Input: part model. Units: mm. Frame: model coordinates. A direction names the side the tool comes from. Coordinates: 2 decimals unless noted, no trailing zeros. Write each loop counter-clockwise with the first axis right and the second up, starting at its lowest first coordinate (ties: lowest second). Pieces come first, ordered by that corner, then holes. Notation, with made-up numbers: M -23.75,82.5 L -0.75,82.5 A16 ccw -0.75,105.5 Z; hole C 15.5,56.5 d3. An arc over 180 degrees is marked long. Answer as a JSON object with one key per item and string values. Group by question number.
from build123d import *

# Parameters (mm, degrees)
BOSS_EXTRUDE1_DEPTH = 13
BOSS_EXTRUDE3_DEPTH = 2.3
BOSS_EXTRUDE4_DEPTH = 2.3
SPLIT1_START        = -4.6
SPLIT1_DEPTH        = 4.6
SKETCH9_W           = 56.929943861
SKETCH9_H           = 73.17042397
BOSS_EXTRUDE5_DEPTH = 34
SKETCH10_W          = 56
SKETCH10_H          = 74
SKETCH10_W_2        = 52
SKETCH10_H_2        = 70
BOSS_EXTRUDE6_DEPTH = 10
SKETCH11_W          = 56
SKETCH11_H          = 74
SKETCH11_W_2        = 52
SKETCH11_H_2        = 70
BOSS_EXTRUDE7_DEPTH = 23
CUT_EXTRUDE1_START  = -74
SKETCH7_R           = 5.3
CUT_EXTRUDE1_DEPTH  = 2
CUT_EXTRUDE2_DEPTH  = 70
CAVITY1_START       = 21.3871
CAVITY1_DEPTH       = 1.6129
SKETCH12_R          = 3.3
CUT_EXTRUDE3_DEPTH  = 2


# Read off the part's stored shape, not the designer's step: Split1, Cavity1
with BuildPart() as part:
    # Sketch1 → Boss-Extrude1 (new body)
    with BuildSketch(Plane(origin=(0, 0, 0), x_dir=(1, 0, 0), z_dir=(0, 1, 0))):
        Polygon((28, 37.2), (-28, 37.2), (-28, -36.8), (28, -36.8), (28, 0), align=None)
        Polygon((26, 0), (26, 35.2), (-26, 35.2), (-26, -34.8), (26, -34.8), align=None, mode=Mode.SUBTRACT)
    extrude(amount=BOSS_EXTRUDE1_DEPTH)


with BuildPart() as body_2:
    # Sketch5 → Boss-Extrude3 (new body)
    with BuildSketch(Plane.XZ):
        with BuildLine():
            Line((-28, 36.8), (28, 36.8))
            Line((28, 36.8), (28, -37.2))
            Line((28, -37.2), (25, -37.2))
            Line((25, -37.2), (25, -9.8))
            ThreePointArc((25, -9.8), (0, 15.2), (-25, -9.8))
            Line((-25, -9.8), (-25, -37.2))
            Line((-25, -37.2), (-28, -37.2))
            Line((-28, -37.2), (-28, 36.8))
        make_face()
    extrude(amount=BOSS_EXTRUDE3_DEPTH)

    # Sketch6 → Boss-Extrude4 (add)
    with BuildSketch(Plane.XZ.offset(2.3)):
        with BuildLine():
            Line((22.7, -37.2), (28, -37.2))
            Line((28, -37.2), (28, 36.8))
            Line((28, 36.8), (-28, 36.8))
            Line((-28, 36.8), (-28, -37.2))
            Line((-28, -37.2), (-22.7, -37.2))
            Line((-22.7, -37.2), (-22.7, -9.8))
            ThreePointArc((-22.7, -9.8), (0, 12.9), (22.7, -9.8))
            Line((22.7, -9.8), (22.7, -37.2))
        make_face()
    extrude(amount=BOSS_EXTRUDE4_DEPTH)

    # Split1 outline → Split1 (cut)
    with BuildSketch(Plane(origin=(0, 0, 0), x_dir=(1, 0, 0), z_dir=(0, 1, 0)).offset(SPLIT1_START)):
        with BuildLine():
            Line((-28, -36.8), (28, -36.8))
            Line((28, -36.8), (28, 37.2))
            Line((28, 37.2), (22.7, 37.2))
            Line((22.7, 37.2), (22.7, 9.8))
            ThreePointArc((22.7, 9.8), (0, -12.9), (-22.7, 9.8))
            Line((-22.7, 9.8), (-22.7, 37.2))
            Line((-22.7, 37.2), (-28, 37.2))
            Line((-28, 37.2), (-28, -36.8))
        make_face()
    extrude(amount=SPLIT1_DEPTH, mode=Mode.SUBTRACT)


with BuildPart() as body_2_2:
    # Sketch9 → Boss-Extrude5 (new body)
    with BuildSketch(Plane(origin=(0, 13, 0), x_dir=(-1, 0, 0), z_dir=(0, 1, 0))):
        with Locations((0.264790437, -0.308922176)):
            Rectangle(SKETCH9_W, SKETCH9_H)
    extrude(amount=BOSS_EXTRUDE5_DEPTH)


with BuildPart() as part_1:
    add(part.part)

    # Combine1: cut body 2 2
    add(body_2_2.part, mode=Mode.SUBTRACT)

    # Sketch10 → Boss-Extrude6 (add)
    with BuildSketch(Plane(origin=(0, 13, 0), x_dir=(1, 0, 0), z_dir=(0, 1, 0))):
        with Locations((0, 0.2)):
            Rectangle(SKETCH10_W, SKETCH10_H)
        with Locations((0, 0.2)):
            Rectangle(SKETCH10_W_2, SKETCH10_H_2, mode=Mode.SUBTRACT)
    extrude(amount=BOSS_EXTRUDE6_DEPTH)

    # Sketch11 → Boss-Extrude7 (add)
    with BuildSketch(Plane(origin=(0, 23, 0), x_dir=(1, 0, 0), z_dir=(0, 1, 0))):
        with Locations((0, 0.2)):
            Rectangle(SKETCH11_W, SKETCH11_H)
        with Locations((0, 0.2)):
            Rectangle(SKETCH11_W_2, SKETCH11_H_2, mode=Mode.SUBTRACT)
    extrude(amount=-BOSS_EXTRUDE7_DEPTH)

    # Sketch7 → Cut-Extrude1 (cut)
    with BuildSketch(Plane.XY.offset(36.8).offset(CUT_EXTRUDE1_START)):
        with Locations((0, 10)):
            Circle(SKETCH7_R)
    extrude(amount=CUT_EXTRUDE1_DEPTH, mode=Mode.SUBTRACT)

    # Sketch8 → Cut-Extrude2 (cut)
    with BuildSketch(Plane.ZY.offset(28)):
        with BuildLine():
            Line((22.750806662, 6.15), (25.849193338, 6.15))
            ThreePointArc((25.849193338, 6.15), (26.95, 4), (25.849193338, 1.85))
            Line((25.849193338, 1.85), (22.750806662, 1.85))
            ThreePointArc((22.750806662, 1.85), (21.65, 4), (22.750806662, 6.15))
        make_face()
        with BuildLine():
            Line((-25.849193338, 6.15), (-22.750806662, 6.15))
            ThreePointArc((-22.750806662, 6.15), (-21.65, 4), (-22.750806662, 1.85))
            Line((-22.750806662, 1.85), (-25.849193338, 1.85))
            ThreePointArc((-25.849193338, 1.85), (-26.95, 4), (-25.849193338, 6.15))
        make_face()
    extrude(amount=-CUT_EXTRUDE2_DEPTH, mode=Mode.SUBTRACT)

    # Cavity1 outline → Cavity1 (cut)
    with BuildSketch(Plane(origin=(0, 0, 0), x_dir=(1, 0, 0), z_dir=(0, 1, 0)).offset(CAVITY1_START)):
        with BuildLine():
            ThreePointArc((-28, -20.441285249), (-27.241688626, -21.665903715), (-26, -22.395928291))
            Line((-26, -22.395928291), (-26, -20.987393289))
            ThreePointArc((-26, -20.987393289), (-27.027836237, -19.527994439), (-26, -18.068595588))
            Line((-26, -18.068595588), (-26, -16.644860586))
            ThreePointArc((-26, -16.644860586), (-27.241688626, -17.374885162), (-28, -18.599503628))
            Line((-28, -18.599503628), (-28, -20.441285249))
        make_face()
        with BuildLine():
            Line((10.014130308, -34.8), (-10.23489996, -34.8))
            ThreePointArc((-10.23489996, -34.8), (-8.230538078, -35.333645486), (-6.197835522, -35.746397685))
            ThreePointArc((-6.197835522, -35.746397685), (-5.469873643, -36.018934875), (-5.147839508, -36.726394439))
            ThreePointArc((-5.147839508, -36.726394439), (-5.146895808, -36.763245519), (-5.144067255, -36.8))
            Line((-5.144067255, -36.8), (4.758391535, -36.8))
            ThreePointArc((4.758391535, -36.8), (4.761220088, -36.763245519), (4.762163763, -36.726394439))
            ThreePointArc((4.762163763, -36.726394439), (5.049199117, -36.033429793), (5.742163763, -35.746394439))
            Line((5.742163763, -35.746394439), (5.822163763, -35.746394439))
            ThreePointArc((5.822163763, -35.746394439), (7.93260454, -35.337235399), (10.014130308, -34.8))
        make_face()
        with BuildLine():
            Line((-28, 13.400496372), (-28, 11.558714751))
            ThreePointArc((-28, 11.558714751), (-27.241688626, 10.334096285), (-26, 9.604071709))
            Line((-26, 9.604071709), (-26, 11.033690962))
            ThreePointArc((-26, 11.033690962), (-26.997836237, 12.482005561), (-26, 13.930320161))
            Line((-26, 13.930320161), (-26, 15.355139414))
            ThreePointArc((-26, 15.355139414), (-27.241688626, 14.625114838), (-28, 13.400496372))
        make_face()
        with BuildLine():
            Line((26, -21.24169048), (26, -22.661132164))
            ThreePointArc((26, -22.661132164), (27.243136742, -21.927868824), (28, -20.698957885))
            Line((28, -20.698957885), (28, -18.873830992))
            ThreePointArc((28, -18.873830992), (27.243136742, -17.644920054), (26, -16.911656713))
            Line((26, -16.911656713), (26, -18.334298397))
            ThreePointArc((26, -18.334298397), (27.012163763, -19.787994439), (26, -21.24169048))
        make_face()
        with BuildLine():
            ThreePointArc((26, 9.338867836), (27.243136742, 10.072131176), (28, 11.301042115))
            Line((28, 11.301042115), (28, 13.126169008))
            ThreePointArc((28, 13.126169008), (27.243136742, 14.355079946), (26, 15.088343287))
            Line((26, 15.088343287), (26, 13.682945544))
            ThreePointArc((26, 13.682945544), (27.032163763, 12.222005562), (26, 10.761065579))
            Line((26, 10.761065579), (26, 9.338867836))
        make_face()
    extrude(amount=CAVITY1_DEPTH, mode=Mode.SUBTRACT)

    # Sketch12 → Cut-Extrude3 (cut)
    with BuildSketch(Plane(origin=(0, 23, 0), x_dir=(1, 0, 0), z_dir=(0, 1, 0))):
        with Locations((-25.144836237, 12.479605561)):
            Circle(SKETCH12_R)
        with Locations((25.142163763, 12.213605561)):
            Circle(SKETCH12_R)
        with Locations((25.142163763, -19.786394439)):
            Circle(SKETCH12_R)
        with Locations((-25.144836237, -19.520394439)):
            Circle(SKETCH12_R)
        with BuildLine():
            Line((-5.144067255, -36.8), (4.758391535, -36.8))
            Line((4.758391535, -36.8), (5.062163763, -36.8))
            Line((5.062163763, -36.8), (5.062163763, -36.726394439))
            ThreePointArc((5.062163763, -36.726394439), (5.261331152, -36.245561827), (5.742163763, -36.046394439))
            Line((5.742163763, -36.046394439), (5.870241965, -36.042516857))
            ThreePointArc((5.870241965, -36.042516857), (8.935204114, -35.405039737), (11.932081344, -34.5))
            Line((11.932081344, -34.5), (-12.110811403, -34.5))
            ThreePointArc((-12.110811403, -34.5), (-9.196992953, -35.402634382), (-6.215562743, -36.047739555))
            ThreePointArc((-6.215562743, -36.047739555), (-5.68493716, -36.228763375), (-5.447661294, -36.736733155))
            Line((-5.447661294, -36.736733155), (-5.447661294, -36.8))
            Line((-5.447661294, -36.8), (-5.144067255, -36.8))
        make_face()
    extrude(amount=-CUT_EXTRUDE3_DEPTH, mode=Mode.SUBTRACT)


solid = part_1.part
Q1. Draft query along Y for faces 1 (the flat face through (-26, 11, 0)), 2 (the flat face through (-27, 23, 3)), 3 (the cylindrical face through (-27.01, 4.04, 26.95)). Return one class per face: released by +Y, released by -Y, zero draft, split by the parting line, or undercut.
Q2. Pin query (flat end, axial travel): pin 1 Ø1.6 at (x, z) = (-27, 20) entering from +Y. Return the tip coordinate at first contact, or that it passes through.
Q3. Line query: line 1 (Z direction, x = 16.5, y = 3); line 2 (X direction, y = 2.25, z = -18.5); line 3 (Y direction, x = 0, z = -36). Output: solid intervals per line, ascending. Write a range as from..to.
Q4. Section C-C, the plane x = 18. Return the cut outline in (y, z), and give its area (3 significant figures).
Q5. Section A-A, the plane x = 0. Return the cut outline in (y, z).
Q6. Access query for faces 4 (the flat face through (0, 16, -35.2)), 5 (the flat face through (-27, 1.85, 24)), 6 (the cylindrical face through (-27.2, 22, 22.1)). Directions: +Z, -Z, +X, -X, +Y, -Y. A direction counts if a zero-diameter tool reaches every point of the face in a straight line with its end or side. Return the directions, or none.
Q7. Section D-D, the plane y = 10. Return the cut outline in (x, z).
Q8. Section B-B, the plane z = 29.5. Return the cut outline in (x, y).
Filled in:
{
 "1": {"face 1": "zero draft", "face 2": "released by +Y", "face 3": "undercut"},
 "2": {"pin 1": "y = 21"},
 "3": {"line 1": "-37.2..-35.2, 34.8..36.8", "line 2": "-28..-26, 26..28", "line 3": "0..4.7, 15.3..23"},
 "4": {"outline": "M 0,-37.2 L 23,-37.2 L 23,-35.2 L 0,-35.2 Z; M 0,34.8 L 23,34.8 L 23,36.8 L 0,36.8 Z", "area": "92.0 mm^2"},
 "5": {"outline": "M 0,-37.2 L 4.7,-37.2 L 4.7,-35.2 L 0,-35.2 Z; M 0,34.8 L 21,34.8 L 21,36.8 L 0,36.8 Z; M 15.3,-37.2 L 23,-37.2 L 23,-35.2 L 15.3,-35.2 Z"},
 "6": {"face 4": "+Y, -Y", "face 5": "+X, -X", "face 6": "+Y"},
 "7": {"outline": "M -28,-37.2 L -5.3,-37.2 L -5.3,-35.2 L -26,-35.2 L -26,34.8 L 26,34.8 L 26,-35.2 L 5.3,-35.2 L 5.3,-37.2 L 28,-37.2 L 28,36.8 L -28,36.8 Z"},
 "8": {"outline": "M -28,0 L -26,0 L -26,23 L -28,23 Z; M 26,0 L 28,0 L 28,23 L 26,23 Z"}
}
